Here's how the part is built. I have some questions about the finished solid (model axes, mm). Coordinates: 2 decimals unless noted, no trailing zeros. Loops run counter-clockwise (first coordinate to the right, second up) from the corner with the lowest first, then second, coordinate; pieces in that order, holes last. Notation, with made-up numbers: M 36.25,-39 L 58.25,-39 A26 cw 58.25,-13 Z; hole C 45.5,66.5 d9. An arc over 180 degrees is marked long. Use one line per item in the form item = value. Start each with the question number.
(1) Imagine slicing it at B-B, the plane z = -157.5. Please give me the cut outline in (x, y), and give its area (3 significant figures).
(2) Please list where these lines run through material, in increasing order: L1, parallel to Z at x = -286, y = 6.25; L2, parallel to X at y = 13.75, z = -157.5.
(3) Imagine slicing it at A-A, the plane x = -106. Please give me the cut outline in (y, z), and give its area (3 significant figures).
(4) Will these pins go through, and if not, where does the flat tip stop? P1, Ø5.5, axis at x = -262.5, y = 11.5, coming from the -Z side; P2, Ø3, axis at y = 9, z = -261, coming from the -X side; P3, Ø9, axis at y = 10, z = -469, coming from the +X side.
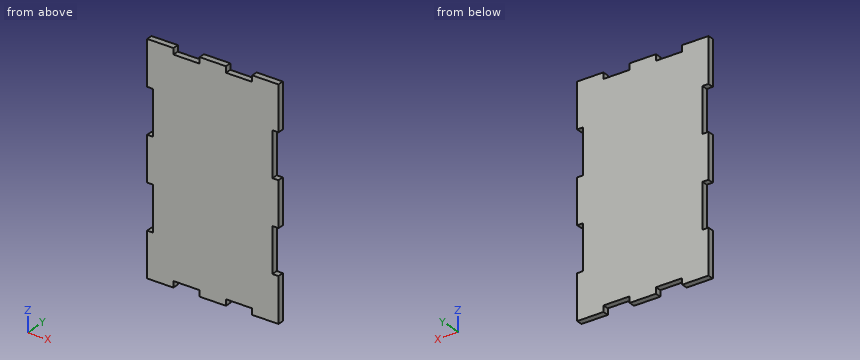
Autodesk Inventor part; units mm, degrees
ref_plane "YZ Plane" through (0, 0, 0) normal (1, 0, 0) x (0, 1, 0)
ref_plane "XZ Plane" through (0, 0, 0) normal (0, 1, 0) x (-1, 0, 0)
ref_plane "XY Plane" through (0, 0, 0) normal (0, 0, 1) x (1, 0, 0)
sketch "Sketch1" plane through (0, 0, 0) normal (0, 1, 0) x (-1, 0, 0)
  line L0 (0, -132) -> (18, -132)
  line L1 (0, -264) -> (18, -264)
  line L2 (0, -396) -> (18, -396)
  line L3 (0, -528) -> (18, -528)
  line L4 (390, -132) -> (372, -132)
  line L5 (390, -264) -> (372, -264)
  line L6 (390, -396) -> (372, -396)
  line L7 (390, -528) -> (372, -528)
  line L8 (0, -132) -> (0, 0)
  line L9 (0, -660) -> (0, -528)
  line L10 (0, -396) -> (0, -264)
  line L11 (390, 0) -> (390, -132)
  line L12 (390, -264) -> (390, -396)
  line L13 (390, -528) -> (390, -660)
  line L14 (372, -132) -> (372, -264)
  line L15 (372, -396) -> (372, -528)
  line L16 (18, -396) -> (18, -528)
  line L17 (18, -132) -> (18, -264)
  line L18 (78, 0) -> (78, -18)
  line L19 (156, 0) -> (156, -18)
  line L20 (234, 0) -> (234, -18)
  line L21 (312, 0) -> (312, -18)
  line L22 (78, -642) -> (78, -660)
  line L23 (156, -642) -> (156, -660)
  line L24 (234, -642) -> (234, -660)
  line L25 (312, -642) -> (312, -660)
  line L26 (0, 0) -> (78, 0)
  line L27 (156, 0) -> (234, 0)
  line L28 (312, 0) -> (390, 0)
  line L29 (312, -18) -> (234, -18)
  line L30 (156, -18) -> (78, -18)
  line L31 (390, -660) -> (312, -660)
  line L32 (234, -660) -> (156, -660)
  line L33 (78, -660) -> (0, -660)
  line L34 (312, -642) -> (234, -642)
  line L35 (156, -642) -> (78, -642)
  dimension "d0" = 660
  dimension "d1" = 390
  dimension "d7" = 132
  dimension "d8" = 132
  dimension "d9" = 132
  dimension "d12" = 132
  dimension "d13" = 132
  dimension "d14" = 132
  dimension "d16" = 18
  dimension "d17" = 18
  dimension "d18" = 18
  dimension "d19" = 18
  dimension "d20" = 18
  dimension "d21" = 18
  dimension "d22" = 18
  dimension "d23" = 18
  dimension "d24" = 78
  dimension "d25" = 78
  dimension "d26" = 78
  dimension "d27" = 78
  dimension "d28" = 78
  dimension "d29" = 78
  dimension "d30" = 78
  dimension "d31" = 18
  dimension "d32" = 18
  dimension "d33" = 18
  dimension "d34" = 18
  dimension "d35" = 18
  dimension "d36" = 18
  dimension "d37" = 18
  dimension "d38" = 18
  dimension "d39" = 132
  dimension "d40" = 132
extrude "Extrusion1" add sketch "Sketch1" along normal blind 18
properties part number "cajon abajo"
Answer:
q1.outline = M -372,0 L -18,0 L -18,18 L -372,18 Z
q1.area = 6,370 mm²
q2.L1 = -642 to -18
q2.L2 = -372 to -18
q3.outline = M 0,-642 L 18,-642 L 18,-18 L 0,-18 Z
q3.area = 11,200 mm²
q4.P1 = -642
q4.P2 = -372
q4.P3 = -18
